Verification items for the finished model (mm, model axes). Face numbers are marked on the shaded views. A direction names the side the tool comes from. Round coordinates to 2 decimals unless told otherwise and drop trailing zeros. Loops run counter-clockwise (first coordinate to the right, second up) from the corner with the lowest first, then second, coordinate; pieces in that order, holes last. Notation, with made-up numbers: (-6, -23) -> (19, -23) arc R13 ccw to (19, -8) -> close; hole circle Ø9 at (18.25, 11). An arc over 180 degrees is marked (long way). Write item = value, one per line.
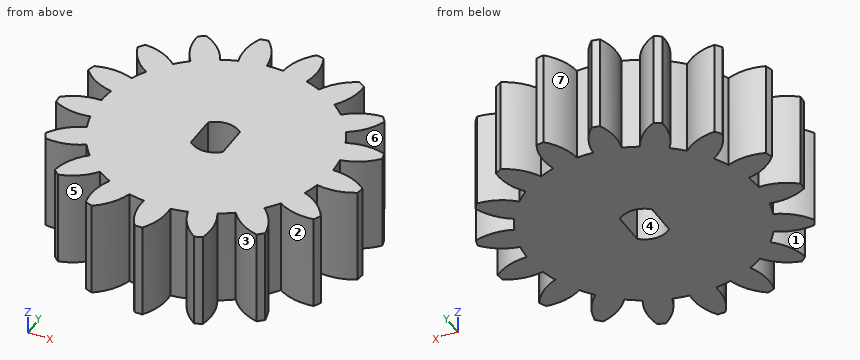
```python
from build123d import *

# Parameters (mm, degrees)
SALIENTE_EXTRUIR1_DEPTH    = 12
CORTAR_EXTRUIR1_DEPTH      = 30.323828441
CORTAR_EXTRUIR1_DEPTH_BACK = 30.323828441


with BuildPart() as part:
    # Croquis2 → Saliente-Extruir1 (new body)
    with BuildSketch(Plane.XY):
        with BuildLine():
            ThreePointArc((-18.403869346, 4.841504781), (-16.568558398, 3.287756261), (-14.307209233, 2.469953906))
            ThreePointArc((-14.307209233, 2.469953906), (-14.437149822, 1.457270995), (-14.495501716, 0.437954415))
            ThreePointArc((-14.495501716, 0.437954415), (-16.868617902, 0.049598518), (-18.958179734, -1.140456979))
            ThreePointArc((-18.958179734, -1.140456979), (-18.91894935, -1.633626778), (-18.86689205, -2.125607989))
            ThreePointArc((-18.86689205, -2.125607989), (-16.594236855, -2.91144455), (-14.190167272, -2.857128995))
            ThreePointArc((-14.190167272, -2.857128995), (-13.94551, -3.848367642), (-13.631701901, -4.819931181))
            ThreePointArc((-13.631701901, -4.819931181), (-15.70427651, -6.039330716), (-17.22283726, -7.903861216))
            ThreePointArc((-17.22283726, -7.903861216), (-17.008102536, -8.349556708), (-16.781836437, -8.789510259))
            ThreePointArc((-16.781836437, -8.789510259), (-14.378771672, -8.70130328), (-12.15666459, -7.782205431))
            ThreePointArc((-12.15666459, -7.782205431), (-11.570451778, -8.618127541), (-10.926865208, -9.410723))
            ThreePointArc((-10.926865208, -9.410723), (-12.418985555, -11.296479508), (-13.161455179, -13.583669836))
            ThreePointArc((-13.161455179, -13.583669836), (-12.800217229, -13.921697376), (-12.430300822, -14.250205101))
            ThreePointArc((-12.430300822, -14.250205101), (-10.221373699, -13.299867423), (-8.481336993, -11.640116539))
            ThreePointArc((-8.481336993, -11.640116539), (-7.63273993, -12.207826199), (-6.746294822, -12.714409169))
            ThreePointArc((-6.746294822, -12.714409169), (-7.456441785, -15.011840784), (-7.322545645, -17.412793212))
            ThreePointArc((-7.322545645, -17.412793212), (-6.863591658, -17.597500307), (-6.399984203, -17.770195419))
            ThreePointArc((-6.399984203, -17.770195419), (-4.68352257, -16.086075411), (-3.660557838, -13.909830045))
            ThreePointArc((-3.660557838, -13.909830045), (-2.664184259, -14.132654921), (-1.654599937, -14.284808564))
            ThreePointArc((-1.654599937, -14.284808564), (-1.486864235, -16.683634417), (-0.494685747, -18.874087015))
            ThreePointArc((-0.494685747, -18.874087015), (0, -18.880527949), (0.494685747, -18.874087015))
            ThreePointArc((0.494685747, -18.874087015), (1.486864235, -16.683634417), (1.654599937, -14.284808564))
            ThreePointArc((1.654599937, -14.284808564), (2.664184259, -14.132654921), (3.660557838, -13.909830045))
            ThreePointArc((3.660557838, -13.909830045), (4.68352257, -16.086075411), (6.399984203, -17.770195419))
            ThreePointArc((6.399984203, -17.770195419), (6.863591658, -17.597500307), (7.322545645, -17.412793212))
            ThreePointArc((7.322545645, -17.412793212), (7.456441785, -15.011840784), (6.746294822, -12.714409169))
            ThreePointArc((6.746294822, -12.714409169), (7.63273993, -12.207826199), (8.481336993, -11.640116539))
            ThreePointArc((8.481336993, -11.640116539), (10.221373699, -13.299867423), (12.430300822, -14.250205101))
            ThreePointArc((12.430300822, -14.250205101), (12.800217229, -13.921697376), (13.161455179, -13.583669836))
            ThreePointArc((13.161455179, -13.583669836), (12.418985555, -11.296479508), (10.926865208, -9.410723))
            ThreePointArc((10.926865208, -9.410723), (11.570451778, -8.618127541), (12.15666459, -7.782205431))
            ThreePointArc((12.15666459, -7.782205431), (14.378771672, -8.70130328), (16.781836437, -8.789510259))
            ThreePointArc((16.781836437, -8.789510259), (17.008102536, -8.349556708), (17.22283726, -7.903861216))
            ThreePointArc((17.22283726, -7.903861216), (15.70427651, -6.039330716), (13.631701901, -4.819931181))
            ThreePointArc((13.631701901, -4.819931181), (13.94551, -3.848367642), (14.190167272, -2.857128995))
            ThreePointArc((14.190167272, -2.857128995), (16.594236855, -2.91144455), (18.86689205, -2.125607989))
            ThreePointArc((18.86689205, -2.125607989), (18.91894935, -1.633626778), (18.958179734, -1.140456979))
            ThreePointArc((18.958179734, -1.140456979), (16.868617902, 0.049598518), (14.495501716, 0.437954415))
            ThreePointArc((14.495501716, 0.437954415), (14.437149822, 1.457270995), (14.307209233, 2.469953906))
            ThreePointArc((14.307209233, 2.469953906), (16.568558398, 3.287756261), (18.403869346, 4.841504781))
            ThreePointArc((18.403869346, 4.841504781), (18.27468722, 5.319068863), (18.133114985, 5.793107654))
            ThreePointArc((18.133114985, 5.793107654), (15.754758974, 6.147964559), (13.401603701, 5.652827203))
            ThreePointArc((13.401603701, 5.652827203), (12.978972561, 6.582232472), (12.491983309, 7.479591209))
            ThreePointArc((12.491983309, 7.479591209), (14.305204321, 9.059062734), (15.455302108, 11.170880865))
            ThreePointArc((15.455302108, 11.170880865), (15.162327318, 11.569530143), (14.859072577, 11.960416361))
            ThreePointArc((14.859072577, 11.960416361), (12.513132546, 11.432149282), (10.497744846, 10.120389716))
            ThreePointArc((10.497744846, 10.120389716), (9.767913137, 10.834362342), (8.989645818, 11.495203635))
            ThreePointArc((8.989645818, 11.495203635), (10.109853132, 13.623027949), (10.419410679, 16.007702951))
            ThreePointArc((10.419410679, 16.007702951), (10.002211095, 16.27359763), (9.578230081, 16.528539926))
            ThreePointArc((9.578230081, 16.528539926), (7.58153823, 15.188494259), (6.17610738, 13.237272882))
            ThreePointArc((6.17610738, 13.237272882), (5.237642918, 13.639386906), (4.273206846, 13.974460476))
            ThreePointArc((4.273206846, 13.974460476), (4.549110257, 16.363263115), (3.976320102, 18.698731414))
            ThreePointArc((3.976320102, 18.698731414), (3.491240839, 18.795960945), (3.003794538, 18.880527949))
            ThreePointArc((3.003794538, 18.880527949), (1.626015166, 16.909684287), (1.020352389, 14.582524357))
            ThreePointArc((1.020352389, 14.582524357), (0, 14.618472051), (-1.020352389, 14.582524357))
            ThreePointArc((-1.020352389, 14.582524357), (-1.626015166, 16.909684287), (-3.003794538, 18.880527949))
            ThreePointArc((-3.003794538, 18.880527949), (-3.491240839, 18.795960945), (-3.976320102, 18.698731414))
            ThreePointArc((-3.976320102, 18.698731414), (-4.549110257, 16.363263115), (-4.273206846, 13.974460476))
            ThreePointArc((-4.273206846, 13.974460476), (-5.237642918, 13.639386906), (-6.17610738, 13.237272882))
            ThreePointArc((-6.17610738, 13.237272882), (-7.58153823, 15.188494259), (-9.578230081, 16.528539926))
            ThreePointArc((-9.578230081, 16.528539926), (-10.002211095, 16.27359763), (-10.419410679, 16.007702951))
            ThreePointArc((-10.419410679, 16.007702951), (-10.109853132, 13.623027949), (-8.989645818, 11.495203635))
            ThreePointArc((-8.989645818, 11.495203635), (-9.767913137, 10.834362342), (-10.497744846, 10.120389716))
            ThreePointArc((-10.497744846, 10.120389716), (-12.513132546, 11.432149282), (-14.859072577, 11.960416361))
            ThreePointArc((-14.859072577, 11.960416361), (-15.162327318, 11.569530143), (-15.455302108, 11.170880865))
            ThreePointArc((-15.455302108, 11.170880865), (-14.305204321, 9.059062734), (-12.491983309, 7.479591209))
            ThreePointArc((-12.491983309, 7.479591209), (-12.978972561, 6.582232472), (-13.401603701, 5.652827203))
            ThreePointArc((-13.401603701, 5.652827203), (-15.754758974, 6.147964559), (-18.133114985, 5.793107654))
            ThreePointArc((-18.133114985, 5.793107654), (-18.27468722, 5.319068863), (-18.403869346, 4.841504781))
        make_face()
    extrude(amount=SALIENTE_EXTRUIR1_DEPTH)

    # Croquis3 → Cortar-Extruir1 (cut, two sides: drawn at the far end of the back side and taken through both)
    with BuildSketch(Plane.XY.offset(12).offset(-CORTAR_EXTRUIR1_DEPTH_BACK)):
        with BuildLine():
            Line((-2, -2.1), (-2, 2.1))
            ThreePointArc((-2, 2.1), (0, 2.9), (2, 2.1))
            Line((2, 2.1), (2, -2.1))
            ThreePointArc((2, -2.1), (0, -2.9), (-2, -2.1))
        make_face()
    extrude(amount=CORTAR_EXTRUIR1_DEPTH + CORTAR_EXTRUIR1_DEPTH_BACK, mode=Mode.SUBTRACT)


solid = part.part
```
(1) Sectioned sample at B-B, the plane y = 12.5. Record the cut outline in (x, z), and give its area (3 significant figures).
Filled sheet:
outline = (-9.64, 0) -> (9.64, 0) -> (9.64, 12) -> (-9.64, 12) -> close
area = 231 mm2
(2) Sectioned sample at A-A, the plane y = 1. Record the cut outline in (x, z).
Filled sheet:
outline = (-14.47, 0) -> (-2, 0) -> (-2, 12) -> (-14.47, 12) -> close; (2, 0) -> (14.47, 0) -> (14.47, 12) -> (2, 12) -> close
(3) Draft check along Y on the marked faces 4, 5, 6 and 7. Enter one of: released by +Y, released by -Y, zero draft, split by the parting line, or undercut.
Filled sheet:
face_4 = undercut
face_5 = released by -Y
face_6 = undercut
face_7 = released by +Y
(4) Go/stop test with flat-tipped pins: pin 1 Ø5 at (y, z) = (1, 6.5) entering from +X; pin 2 Ø2 at (y, z) = (0.5, 4) entering from -X; pin 3 Ø1.5 at (x, z) = (8.5, 6) entering from +Y; pin 4 Ø5 at (y, z) = (7.5, 2) entering from -X. Record where each tip stops, or that it passes through.
Filled sheet:
pin_1 = 18.96
pin_2 = -18.05
pin_3 = 16.37
pin_4 = -18.36
(5) Material ranges on probe 1 along Y at (x, z) = (-16, 8.25); probe 2 along X at (y, z) = (-8, 3); probe 3 along Y at (x, z) = (-12, 1.75), recorded low to high. Write a range as from..to.
Filled sheet:
probe_1 = -8.85..-6.31, -2.98..0.29, 2.99..6.15
probe_2 = -17.18..-12.52, -12.01..12.01, 12.52..17.18
probe_3 = -14.14..-10.61, -8.02..11.19
(6) Set-up check for the marked faces 1, 2 and 3: record each of +Z, -Z, +X, -X, +Y, -Y from which the full face is reachable in a straight line by a thin tool's end or side.
Filled sheet:
face_1 = +Z, -Z, -X
face_2 = +Z, -Z
face_3 = +Z, -Z, -Y
